Input: dimensioned drawing with shaded views. Units: mm. Origin: part minimum x, y, z. A direction names the side the tool comes from. Give positions to 0.01 mm unless a question says otherwise; leave off trailing zeros. Order: outer loops, then holes, each group sorted by start corner. A loop starts at its lowest first (then second) coordinate and runs counter-clockwise, first axis right, second up.
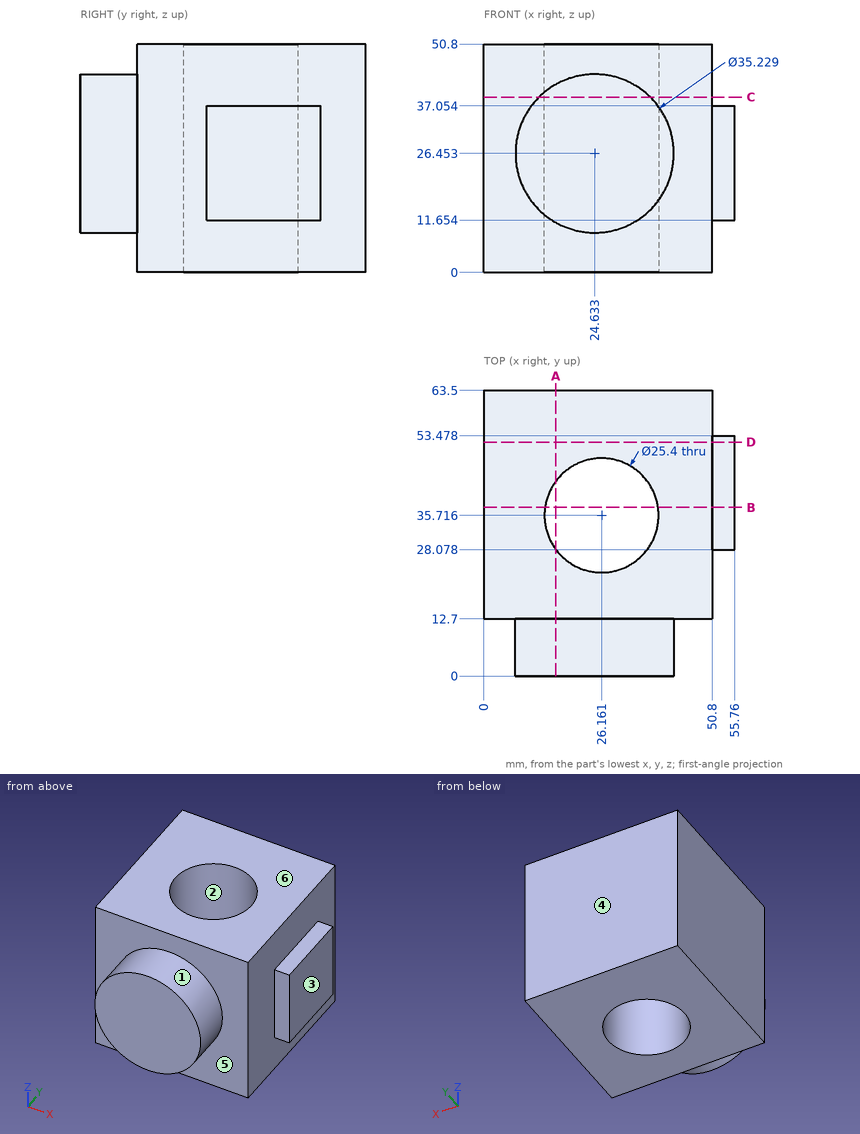
1) Pin query (flat end, axial travel): pin 1 (4 mm diameter, centred on x = 44.5, z = 23.5, fed in from -Y); pin 2 (2.5 mm diameter, centred on x = 53.5, z = 22, fed in from -Y); pin 3 (4 mm diameter, centred on x = 53.5, y = 39.5, fed in from -Z). Return the tip coordinate at first contact, or that it passes through.
Report:
pin 1: stops at y = 12.7
pin 2: stops at y = 28.08
pin 3: stops at z = 11.65
2) Reachability of the marked faces 5 and 6 from +Z, -Z, +X, -X, +Y, -Y: full face, straight path, thin tool, end or side. Return the list, or none.
Report:
face 5: -Y
face 6: +Z, +X, -X, +Y, -Y
3) Section query C-C, the plane z = 39. Return the cut outline in (x, y), and give its area (3 significant figures).
Report:
outline: (0, 12.7) - (12.27, 12.7) - (12.27, 0) - (37, 0) - (37, 12.7) - (50.8, 12.7) - (50.8, 63.5) - (0, 63.5) - close; hole circle Ø25.4 at (26.16, 35.72)
area: 2,390 mm2
4) Section query B-B, the plane y = 37.5. Return the cut outline in (x, z) (1 decimal).
Report:
outline: (0, 0) - (13.6, 0) - (13.6, 50.8) - (0, 50.8) - close; (38.7, 0) - (50.8, 0) - (50.8, 11.7) - (55.8, 11.7) - (55.8, 37.1) - (50.8, 37.1) - (50.8, 50.8) - (38.7, 50.8) - close
5) Material intervals for L1, parallel to Y at x = 44, z = 48.5; L2, parallel to X at y = 44.5, z = 45 (1 decimal); L3, parallel to Y at x = 32, z = 35.5 (1 decimal), sorted ascending.
Report:
L1: y = 12.7 to 63.5
L2: x = 0 to 17, 35.3 to 50.8
L3: y = 0 to 24.4, 47 to 63.5
6) Section query D-D, the plane y = 52. Return the cut outline in (x, z) (1 decimal), and give its area (3 significant figures).
Report:
outline: (0, 0) - (50.8, 0) - (50.8, 11.7) - (55.8, 11.7) - (55.8, 37.1) - (50.8, 37.1) - (50.8, 50.8) - (0, 50.8) - close
area: 2,710 mm2
7) Draft query along X for the marked faces 1, 2, 3 and 4. Return one class per face: +X half, -X half, draft (parallel to the pull), parting line (faces both ways), or undercut.
Report:
face 1: parting line
face 2: undercut
face 3: +X half
face 4: draft
8) Section query A-A, the plane x = 16. Return the cut outline in (y, z) (1 decimal), and give its area (3 significant figures).
Report:
outline: (0, 11.1) - (12.7, 11.1) - (12.7, 0) - (28.1, 0) - (28.1, 50.8) - (12.7, 50.8) - (12.7, 41.8) - (0, 41.8) - close; (43.3, 0) - (63.5, 0) - (63.5, 50.8) - (43.3, 50.8) - close
area: 2,200 mm2
